Geometry check sheet. Reference: drawing and pictorial views, mm from the part's lowest x, y, z. A direction names the side the tool comes from. Round coordinates to 2 decimals unless told otherwise and drop trailing zeros. Loops run counter-clockwise (first coordinate to the right, second up) from the corner with the lowest first, then second, coordinate; pieces in that order, holes last. Notation, with made-up numbers: M -31,-19.75 L -19,-19.75 A25 cw -19,13.25 Z; hole C 60,21 d5. An arc over 180 degrees is marked long. One line per question, with ' | ' between items. Start each with the question number.
(1) Draft check along Y on the marked faces 1, 2 and 3. Enter one of: +Y half, -Y half, draft (parallel to the pull), parting line (faces both ways), or undercut.
(2) Tool access check on the marked faces 4, 5 and 6. Record the directions out of +Z, -Z, +X, -X, +Y, -Y that give a thin tool (end or side, any length) a straight path to the whole face; none if there is none.
(3) Thickness scan on probe 1 along X at (y, z) = (2, 5); probe 2 along X at (y, z) = (3.5, 4.5); probe 3 along Y at (x, z) = (8.75, 4.5). Record the ranges inside material, lowest first. Write a range as [from, to].
(4) Go/stop test with flat-tipped pins: P1, Ø1.5, axis at x = 3.5, y = 2, coming from the +Z side; P2, Ø1.5, axis at y = 4, z = 3.5, coming from the -X side; P3, Ø1.5, axis at x = 6.5, y = 3, coming from the -Z side. Record where each tip stops, or that it passes through.
(5) Section check A-A (x = 11.75). Record the boundary of the cut face in (y, z), and give its area (3 significant figures).
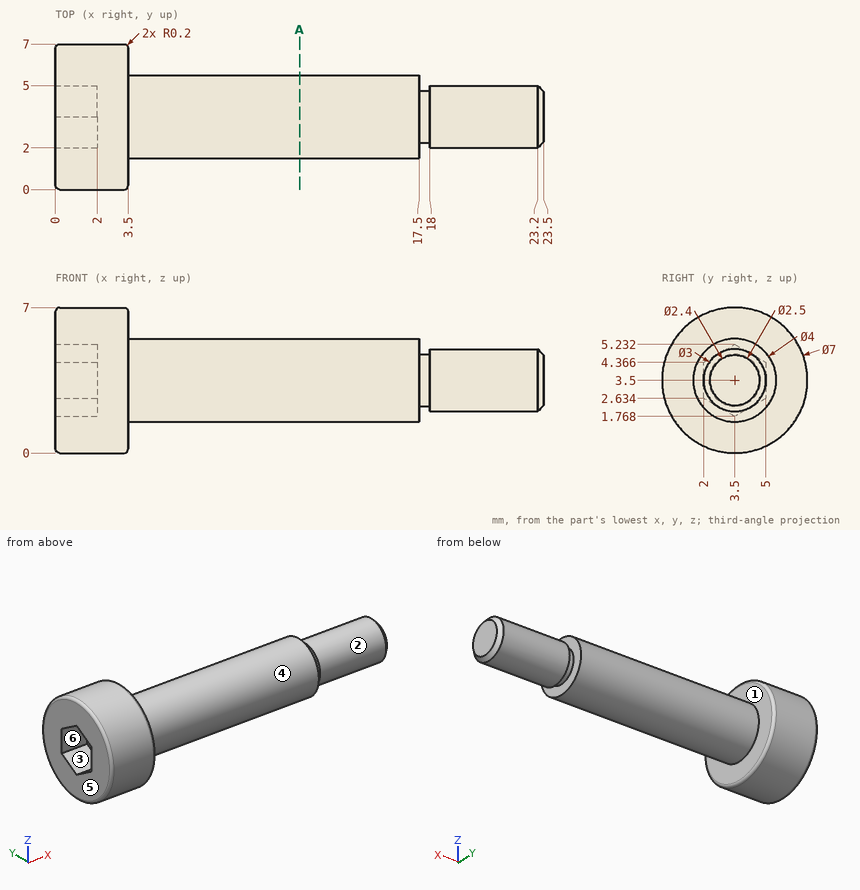
The answers:
1) face 1: draft | face 2: parting line | face 3: undercut
2) face 4: +X | face 5: +Z, -Z, -X, +Y, -Y | face 6: -X
3) probe 1: [0, 3.5] | probe 2: [2, 23.5] | probe 3: [1.77, 5.23]
4) P1: z = 6.91 | P2: x = 2 | P3: z = 1.5
5) outline: C 3.5,3.5 d4 | area: 12.6 mm²
